Build history of the part. All positions in model axes, mm. A direction names the side the tool comes from. Coordinates: 2 decimals unless noted, no trailing zeros. Order: outer loops, then holes, each group sorted by start corner. A loop starts at its lowest first (then second) coordinate and runs counter-clockwise, first axis right, second up. Notation, with made-up numbers: (54, 61.5) - (86, 61.5) arc R29 ccw to (86, 81.5) - close; hole circle Ø11 at (64, 5). An arc over 180 degrees is marked (long way). Return JSON: item names as keys, results as strings.
from build123d import *

# Parameters (mm, degrees)
SKETCH1_W           = 50.8
SKETCH1_H           = 50.8
SKETCH1_W_2         = 47.625
SKETCH1_H_2         = 47.625
BOSS_EXTRUDE1_DEPTH = 304.8
CUT_EXTRUDE1_DEPTH  = 304.8
SKETCH3_R           = 2.5796875
CUT_EXTRUDE2_DEPTH  = 159
SKETCH4_R           = 9.525
CUT_EXTRUDE3_DEPTH  = 3.175


with BuildPart() as part:
    # Sketch1 → Boss-Extrude1 (new body)
    with BuildSketch(Plane.XY):
        with Locations((-3.936730361, -0.161783439)):
            Rectangle(SKETCH1_W, SKETCH1_H)
        with Locations((-3.936730361, -0.161783439)):
            Rectangle(SKETCH1_W_2, SKETCH1_H_2, mode=Mode.SUBTRACT)
    extrude(amount=BOSS_EXTRUDE1_DEPTH)

    # Sketch2 → Cut-Extrude1 (cut)
    with BuildSketch(Plane(origin=(21.463269639, 0, 0), x_dir=(0, 0, -1), z_dir=(1, 0, 0))):
        Polygon((-280.250738686, -0.161783439), (-283.000369343, 4.600716561), (-288.499630657, 4.600716561), (-291.249261314, -0.161783439), (-288.499630657, -4.924283439), (-283.000369343, -4.924283439), align=None)
    extrude(amount=-CUT_EXTRUDE1_DEPTH, mode=Mode.SUBTRACT)

    # Sketch3 → Cut-Extrude2 (cut)
    with BuildSketch(Plane(origin=(21.463269639, 0, 0), x_dir=(0, 0, -1), z_dir=(1, 0, 0))):
        with Locations(Location((-6.35, 0, 0), (0, 0, 90))):
            Circle(SKETCH3_R)
        with Locations(Location((-19.05, 0, 0), (0, 0, 90))):
            Circle(SKETCH3_R)
    extrude(amount=-CUT_EXTRUDE2_DEPTH, mode=Mode.SUBTRACT)

    # Sketch4 → Cut-Extrude3 (cut)
    with BuildSketch(Plane.ZY.offset(29.336730361)):
        with Locations(Location((286.190661961, 0, 0), (0, 0, 270))):
            Circle(SKETCH4_R)
    extrude(amount=-CUT_EXTRUDE3_DEPTH, mode=Mode.SUBTRACT)


solid = part.part
1. Probe L1, parallel to Z at x = -28.7, y = 0; L2, parallel to Y at x = -23, z = 238; L3, parallel to X at y = -17, z = 217. List the from-to ranges inside material, lowest first.
Check values:
{"L1": "0 to 3.77, 8.93 to 16.47, 21.63 to 276.67, 295.72 to 304.8", "L2": "-25.56 to -23.97, 23.65 to 25.24", "L3": "-29.34 to -27.75, 19.88 to 21.46"}
2. Cut at D-D on z = 63.5. Give the cut face in (x, y), plus the area to 4 significant figures.
Check values:
{"outline": "(-29.34, -25.56) - (21.46, -25.56) - (21.46, 25.24) - (-29.34, 25.24) - close; hole (-27.75, -23.97) - (19.88, -23.97) - (19.88, 23.65) - (-27.75, 23.65) - close", "area": "312.5 mm²"}
3. Cut at A-A on y = -14. Give the cut face in (x, z).
Check values:
{"outline": "(-29.34, 0) - (-27.75, 0) - (-27.75, 304.8) - (-29.34, 304.8) - close; (19.88, 0) - (21.46, 0) - (21.46, 304.8) - (19.88, 304.8) - close"}
4. Cut at C-C on z = 6.35. Give the cut face in (x, y), plus the area to 3 significant figures.
Check values:
{"outline": "(-29.34, -25.56) - (21.46, -25.56) - (21.46, -2.58) - (19.88, -2.58) - (19.88, -23.97) - (-27.75, -23.97) - (-27.75, -2.58) - (-29.34, -2.58) - close; (-29.34, 2.58) - (-27.75, 2.58) - (-27.75, 23.65) - (19.88, 23.65) - (19.88, 2.58) - (21.46, 2.58) - (21.46, 25.24) - (-29.34, 25.24) - close", "area": "296 mm²"}
5. Tool access for faces 4 (the flat face through (-4, 23.651, 150)), 5 (the cylindrical face through (-28.554, 1.24, 295.635)), 6 (the flat face through (21.463, -1, 150)): list every direction of +Z, -Z, +X, -X, +Y, -Y with a clear straight run to the whole face (end or side of a thin tool).
Check values:
{"face 4": "+Z, -Z", "face 5": "-X", "face 6": "+Z, -Z, +X, +Y, -Y"}
6. Drop flat-ended pins along their axis: pin 1 (11.5 mm diameter, centred on y = 0, z = 286.19, fed in from -X); pin 2 (6 mm diameter, centred on x = -16.5, y = 18.5, fed in from -Z). Give the stop position or say it passes through.
Check values:
{"pin 1": "x = 19.88", "pin 2": "through"}
7. Mould opens along Z. For faces 1 (the cylindrical face through (-28.53, -0.56, 3.83)), 2 (the flat face through (-6, -25, 304.8)), 3 (the flat face through (-27.749, 0, 150)) say: pulls with the +Z half, pulls with the -Z half, needs draft (parallel to the pull), parting line crosses it, or undercut.
Check values:
{"face 1": "undercut", "face 2": "pulls with the +Z half", "face 3": "needs draft"}
8. Cut at B-B on x = 15. Give the cut face in (y, z).
Check values:
{"outline": "(-25.56, 0) - (-23.97, 0) - (-23.97, 304.8) - (-25.56, 304.8) - close; (23.65, 0) - (25.24, 0) - (25.24, 304.8) - (23.65, 304.8) - close"}
